from build123d import *

# Parameters (mm, degrees)
BOSS_EXTRUDE1_DEPTH = 35
FILLET1_R           = 10
FILLET2_R           = 10
BOSS_EXTRUDE2_DEPTH = 70
SKETCH4_R           = 5
CUT_EXTRUDE1_DEPTH  = 70


with BuildPart() as part:
    # Sketch1 → Boss-Extrude1 (new body, symmetric)
    with BuildSketch(Plane.XY):
        with BuildLine():
            Line((-75.172413793, -24.310344828), (-75.172413793, 35.689655172))
            Line((-75.172413793, 35.689655172), (-45.172413793, 35.689655172))
            Line((-45.172413793, 35.689655172), (-45.172413793, 5.689655172))
            Line((-45.172413793, 5.689655172), (24.827586207, 5.689655172))
            Line((24.827586207, 5.689655172), (24.827586207, -14.310344828))
            Line((24.827586207, -14.310344828), (42.32758867, -14.310344828))
            ThreePointArc((42.32758867, -14.310344828), (59.827586207, 3.198940398), (77.327583744, -14.310344828))
            Line((77.327583744, -14.310344828), (94.827586207, -14.310344828))
            Line((94.827586207, -14.310344828), (94.827586207, -24.310344828))
            Line((94.827586207, -24.310344828), (69.827586207, -24.310344828))
            Line((69.827586207, -24.310344828), (69.827586207, -14.301059602))
            ThreePointArc((69.827586207, -14.301059602), (59.827586207, -4.301059602), (49.827586207, -14.301059602))
            Line((49.827586207, -14.301059602), (49.827586207, -24.310344828))
            Line((49.827586207, -24.310344828), (-75.172413793, -24.310344828))
        make_face()
    extrude(amount=BOSS_EXTRUDE1_DEPTH, both=True)

    # Fillet1
    fillet1_edges = [part.edges().sort_by_distance(p)[0] for p in [
        (-60.172413793, 35.689655172, 35),
    ]]
    fillet(fillet1_edges, radius=FILLET1_R)

    # Fillet2
    fillet2_edges = [part.edges().sort_by_distance(p)[0] for p in [
        (-60.172413793, 35.689655172, -35),
    ]]
    fillet(fillet2_edges, radius=FILLET2_R)

    # Sketch3 → Boss-Extrude2 (add)
    with BuildSketch(Plane(origin=(-45.172413793, 0, 0), x_dir=(0, 0, -1), z_dir=(1, 0, 0))):
        with BuildLine():
            ThreePointArc((0, 5.689655172), (-17.5, 23.189655172), (-35, 5.689655172))
            Line((-35, 5.689655172), (0, 5.689655172))
        make_face()
        with BuildLine():
            ThreePointArc((35, 5.689655172), (17.5, 23.189655172), (0, 5.689655172))
            Line((0, 5.689655172), (35, 5.689655172))
        make_face()
    extrude(amount=BOSS_EXTRUDE2_DEPTH)

    # Sketch4 → Cut-Extrude1 (cut)
    with BuildSketch(Plane(origin=(24.827586207, 0, 0), x_dir=(0, 0, -1), z_dir=(1, 0, 0))):
        with Locations((-17.5, 5.689655172)):
            Circle(SKETCH4_R)
        with Locations((17.5, 5.689655172)):
            Circle(SKETCH4_R)
    extrude(amount=-CUT_EXTRUDE1_DEPTH, mode=Mode.SUBTRACT)


solid = part.part
The model under review builds one solid part; all positions refer to its coordinate system, in mm. A direction names the side the tool comes from. Coordinates: 2 decimals unless noted, no trailing zeros. Loops run counter-clockwise (first coordinate to the right, second up) from the corner with the lowest first, then second, coordinate; pieces in that order, holes last. Notation, with made-up numbers: (47.5, 29) -> (85.5, 29) arc R16 cw to (85.5, 45) -> close; hole circle Ø2 at (21, -30). An arc over 180 degrees is marked (long way). Use a Markdown table: item, result. Add a question column.
1. Add section A-A on y = -20. Write out the cut boundary in (x, z), plus the area to 3 significant figures.
2. Machinability: for faces 4 (the face through (86, -14.31, 0)), 5 (the face through (24.828, 5, 0)), 6 (the face through (-45.172, 6, 18)), 7 (the face through (69.828, -19, 0)), 8 (the face through (-45.172, 28, 0)), which of the approach directions +Z, -Z, +X, -X, +Y, -Y give a long, thin tool a straight path to every point of the face, cutting with its end or side? Answer none if there is none.
3. To check wall thickness, follow line 1 (Y direction, x = -23.5, z = -17.5); line 2 (X direction, y = -10.5, z = 9); line 3 (Z direction, x = 6.5, y = 4.5). State the ranges of each line that lie inside material, in increasing order.
4. Draft analysis for pull direction Y (two halves, no side actions). For faces 1 (the face through (33, -14.31, 0)), 2 (the face through (-9.682, 9.069, 21.185)), 3 (the face through (49.828, -19, 0)), state which applies: pulls with the +Y half, pulls with the -Y half, needs draft (parallel to the pull), parting line crosses it, or undercut.
5. Add section D-D on z = 17.5. Write out the cut boundary in (x, y), plus the area to 3 significant figures.
6. Add section C-C on z = -27. Write out the cut boundary in (x, y), plus the area to 3 significant figures.
7. Clearance check with flat-ended pins moving along their axes: pin 1 Ø5.5 at (x, z) = (34.5, -11) entering from +Y; pin 2 Ø1 at (y, z) = (21, -4.5) entering from +X; pin 3 Ø8 at (y, z) = (4.5, 16.5) entering from +X. State where each tip first meets the part, or that it passes through.
8. Add section B-B on x = -33. Write out the cut boundary in (y, z).
Returned:
| question | item | result |
|---|---|---|
| 1 | outline | (-75.17, -35) -> (49.83, -35) -> (49.83, 35) -> (-75.17, 35) -> close; (69.83, -35) -> (94.83, -35) -> (94.83, 35) -> (69.83, 35) -> close |
| 1 | area | 10,500 mm² |
| 2 | face 4 | +Z, -Z, +X, +Y |
| 2 | face 5 | +Z, -Z, +Y |
| 2 | face 6 | none |
| 2 | face 7 | +Z, -Z, -Y |
| 2 | face 8 | +X, +Y |
| 3 | line 1 | y = -24.31 to 0.69, 10.69 to 23.19 |
| 3 | line 2 | x = -75.17 to 24.83, 42.75 to 50.58, 69.08 to 76.91 |
| 3 | line 3 | z = -35 to -22.36, -12.64 to 12.64, 22.36 to 35 |
| 4 | face 1 | pulls with the +Y half |
| 4 | face 2 | undercut |
| 4 | face 3 | needs draft |
| 5 | outline | (-75.17, -24.31) -> (49.83, -24.31) -> (49.83, -14.3) arc R10 cw to (69.83, -14.3) -> (69.83, -24.31) -> (94.83, -24.31) -> (94.83, -14.31) -> (77.33, -14.31) arc R17.5 ccw to (42.33, -14.31) -> (24.83, -14.31) -> (24.83, 0.69) -> (-45.17, 0.69) -> (-45.17, 10.69) -> (24.83, 10.69) -> (24.83, 23.19) -> (-45.17, 23.19) -> (-45.17, 35.69) -> (-75.17, 35.69) -> close |
| 5 | area | 5,250 mm² |
| 6 | outline | (-75.17, -24.31) -> (49.83, -24.31) -> (49.83, -14.3) arc R10 cw to (69.83, -14.3) -> (69.83, -24.31) -> (94.83, -24.31) -> (94.83, -14.31) -> (77.33, -14.31) arc R17.5 ccw to (42.33, -14.31) -> (24.83, -14.31) -> (24.83, 20.39) -> (-45.17, 20.39) -> (-45.17, 35.49) -> (-75.17, 35.49) -> close |
| 6 | area | 5,750 mm² |
| 7 | pin 1 | stops at y = -14.31 |
| 7 | pin 2 | stops at x = -45.17 |
| 7 | pin 3 | stops at x = 69.16 |
| 8 | outline | (-24.31, -35) -> (5.69, -35) arc R17.5 ccw to (5.69, 0) arc R17.5 ccw to (5.69, 35) -> (-24.31, 35) -> close; hole circle Ø10 at (5.69, -17.5); hole circle Ø10 at (5.69, 17.5) |
